```python
from build123d import *

# Parameters (mm, degrees)
F0_W      = 41.91
F0_H      = 31.75
F1_DEPTH  = 3.175
F4_DEPTH  = 3.176
F5_W      = 21.082
F5_H      = 18.415
F6_DEPTH  = 3.81
F7_W      = 6.35
F7_H      = 25.4
F8_DEPTH  = 4.064
F9_W      = 6.35
F9_H      = 25.4
F10_DEPTH = 1.651
F11_W     = 33.02
F11_H     = 22.86
F12_DEPTH = 1.27


with BuildPart() as f1:
    # F0 (on Front) → F1 (new body)
    with BuildSketch(Plane.XZ):
        Rectangle(F0_W, F0_H)
    extrude(amount=F1_DEPTH)

    # F3 (on face) → F4 (cut, through all)
    with BuildSketch(Plane.XZ.offset(3.175)):
        with BuildLine():
            ThreePointArc((-8.40026, 15.875), (0, 12.7), (8.40026, 15.875))
            Line((8.40026, 15.875), (-8.40026, 15.875))
        make_face()
    extrude(amount=-F4_DEPTH, mode=Mode.SUBTRACT)

    # F5 (on face) → F6 (join)
    with BuildSketch(Plane.XZ.offset(3.175)):
        with Locations((0, 5.08)):
            Rectangle(F5_W, F5_H)
    extrude(amount=F6_DEPTH)

    # F7 (on face) → F8 (join)
    with BuildSketch(Plane.XZ.offset(3.175)):
        with Locations((15.875, 0)):
            Rectangle(F7_W, F7_H)
    extrude(amount=F8_DEPTH)

    # F9 (on face) → F10 (join)
    with BuildSketch(Plane.XZ.offset(3.175)):
        with Locations((-15.875, 0)):
            Rectangle(F9_W, F9_H)
    extrude(amount=F10_DEPTH)

    # F11 (on face) → F12 (join)
    with BuildSketch(Plane(origin=(0, 0, 0), x_dir=(-1, 0, 0), z_dir=(0, 1, 0))):
        Rectangle(F11_W, F11_H)
    extrude(amount=F12_DEPTH)


solid = f1.part
```
Source: CAD feature listing. Evaluate the final solid. Frame: model axes, mm. A direction names the side the tool comes from. Coordinates: 2 decimals unless noted, no trailing zeros. Loops run counter-clockwise (first coordinate to the right, second up) from the corner with the lowest first, then second, coordinate; pieces in that order, holes last. Notation, with made-up numbers: M -2,40 L 13,40 A19 ccw 13,51 Z; hole C 37,86 d11. An arc over 180 degrees is marked long. Use a Markdown table: item, result. Add a question column.
Q1. Material intervals for L1, parallel to X at y = -3.75, z = -2.5; L2, parallel to Z at x = -0.5, y = 0.5; L3, parallel to Y at x = -4, z = 12 (3 decimals), sorted ascending.
Q2. First-contact query: pin 1 (4.5 mm diameter, centred on y = -5.5, z = -5.5, fed in from +X); pin 2 (3.5 mm diameter, centred on x = 15, y = -5, fed in from -Z); pin 3 (0.5 mm diameter, centred on x = 2, z = 14, fed in from +Y) (3 decimals). Flat tips, straight axial feed; report the tip coordinate or a pass-through.
Q3. Section query D-D, the plane y = -1.75. Return loops of the section in (x, z) (3 decimals).
Q4. Access query for faces 1 (the flat face through (16.51, 1, 0)), 2 (the flat face through (19.05, -5, 0)), 3 (the flat face through (-12.7, -4, 0)). Directions: +Z, -Z, +X, -X, +Y, -Y. A direction counts if a zero-diameter tool reaches every point of the face in a straight line with its end or side. Return the directions, or none.
Q5. Section query B-B, the plane x = -9.5. Return loops of the section in (y, z) (1 decimal), and give its area (3 significant figures).
Q6. Section query A-A, the plane y = -3.75. Return loops of the section in (x, z), and give its area (3 significant figures).
Q7. Section query C-C, the plane z = 2.5. Return loops of the section in (x, y) (3 decimals), and give its area (3 significant figures).
Result:
| question | item | result |
|---|---|---|
| 1 | L1 | x = -19.05 to -12.7, -10.54 to 10.54, 12.7 to 19.05 |
| 1 | L2 | z = -11.43 to 11.43 |
| 1 | L3 | y = -6.985 to 0 |
| 2 | pin 1 | stops at x = 19.05 |
| 2 | pin 2 | stops at z = -12.7 |
| 2 | pin 3 | stops at y = -3.175 |
| 3 | outline | M -20.955,-15.875 L 20.955,-15.875 L 20.955,15.875 L 8.4,15.875 A12.7 cw -8.4,15.875 L -20.955,15.875 Z |
| 4 | face 1 | +Z, -Z, +X, +Y |
| 4 | face 2 | +Z, -Z, +X, -Y |
| 4 | face 3 | +Z, -Z, -Y |
| 5 | outline | M -7,-4.1 L -3.2,-4.1 L -3.2,-15.9 L 0,-15.9 L 0,-11.4 L 1.3,-11.4 L 1.3,11.4 L 0,11.4 L 0,15.9 L -3.2,15.9 L -3.2,14.3 L -7,14.3 Z |
| 5 | area | 200 mm2 |
| 6 | outline | M -19.05,-12.7 L -12.7,-12.7 L -12.7,12.7 L -19.05,12.7 Z; M -10.54,-4.13 L 10.54,-4.13 L 10.54,14.29 L -10.54,14.29 Z; M 12.7,-12.7 L 19.05,-12.7 L 19.05,12.7 L 12.7,12.7 Z |
| 6 | area | 711 mm2 |
| 7 | outline | M -20.955,-3.175 L -19.05,-3.175 L -19.05,-4.826 L -12.7,-4.826 L -12.7,-3.175 L -10.541,-3.175 L -10.541,-6.985 L 10.541,-6.985 L 10.541,-3.175 L 12.7,-3.175 L 12.7,-7.239 L 19.05,-7.239 L 19.05,-3.175 L 20.955,-3.175 L 20.955,0 L 16.51,0 L 16.51,1.27 L -16.51,1.27 L -16.51,0 L -20.955,0 Z |
| 7 | area | 292 mm2 |
